```python
from build123d import *

# Parameters (mm, degrees)
BOSS_EXTRUDE1_DEPTH  = 2.7
SKETCH6_W            = 21.5
SKETCH6_H            = 36
BOSS_EXTRUDE2_DEPTH  = 2
SKETCH7_W            = 18.8
SKETCH7_H            = 11.32703558
CUT_EXTRUDE3_DEPTH   = 2
CUT_EXTRUDE4_DEPTH   = 41.5
SKETCH10_R           = 0.5
CUT_EXTRUDE5_DEPTH   = 41.5
CUT_EXTRUDE15_DEPTH  = 16
FILLET6_R            = 5
BOSS_EXTRUDE6_DEPTH  = 36
CUT_EXTRUDE18_DEPTH  = 1
CUT_EXTRUDE22_DEPTH  = 11.327036
CUT_EXTRUDE23_DEPTH  = 11.327036
BOSS_EXTRUDE10_DEPTH = 3
SKETCH43_W           = 2.3
SKETCH43_H           = 2.67296442
SKETCH43_H_2         = 8
SKETCH45_R           = 0.5
CUT_EXTRUDE26_DEPTH  = 38.82703558
SKETCH47_W           = 3.454078762
SKETCH47_H           = 22.63811533
CUT_EXTRUDE27_DEPTH  = 4
FILLET13_R           = 2
FILLET15_R           = 1
BOSS_EXTRUDE5_DEPTH  = 0.5
FILLET7_R            = 5


with BuildPart() as part:
    # Sketch3 → Boss-Extrude1 (new body)
    with BuildSketch(Plane(origin=(0, 0, 0), x_dir=(0, 0, -1), z_dir=(1, 0, 0))):
        with BuildLine():
            Line((0, 0), (45, 0))
            ThreePointArc((45, 0), (22.5, 6.928108612), (0, 0))
        make_face()
    extrude(amount=BOSS_EXTRUDE1_DEPTH)

    # Sketch6 → Boss-Extrude2 (add)
    with BuildSketch(Plane.XZ):
        with Locations((10.75, -22.5)):
            Rectangle(SKETCH6_W, SKETCH6_H)
    extrude(amount=BOSS_EXTRUDE2_DEPTH)

    # Sketch7 → Cut-Extrude3 (cut)
    with BuildSketch(Plane(origin=(0, 0, 0), x_dir=(1, 0, 0), z_dir=(0, 1, 0))):
        with Locations((12.1, 32.16351779)):
            Rectangle(SKETCH7_W, SKETCH7_H)
        with Locations((12.1, 12.83648221)):
            Rectangle(SKETCH7_W, SKETCH7_H)
    extrude(amount=-CUT_EXTRUDE3_DEPTH, mode=Mode.SUBTRACT)

    # Sketch8 → Cut-Extrude4 (cut, through all)
    with BuildSketch(Plane(origin=(0, 0, -40.5), x_dir=(-1, 0, 0), z_dir=(0, 0, -1))):
        with BuildLine():
            ThreePointArc((-21.5, -1), (-21.207106781, -0.292893219), (-20.5, 0))
            Line((-20.5, 0), (-21.5, 0))
            Line((-21.5, 0), (-21.5, -1))
        make_face()
        with BuildLine():
            ThreePointArc((-20.5, -2), (-21.207106781, -1.707106781), (-21.5, -1))
            Line((-21.5, -1), (-21.5, -2))
            Line((-21.5, -2), (-20.5, -2))
        make_face()
    extrude(amount=-CUT_EXTRUDE4_DEPTH, mode=Mode.SUBTRACT)

    # Sketch10 → Cut-Extrude5 (cut, through all)
    with BuildSketch(Plane(origin=(0, 0, -40.5), x_dir=(-1, 0, 0), z_dir=(0, 0, -1))):
        with Locations((-20.5, -1)):
            Circle(SKETCH10_R)
    extrude(amount=-CUT_EXTRUDE5_DEPTH, mode=Mode.SUBTRACT)

    # Sketch23 → Cut-Extrude15 (cut)
    with BuildSketch(Plane(origin=(0, 0, 0), x_dir=(1, 0, 0), z_dir=(0, 1, 0))):
        Polygon((11.878000054, 16.672665213), (21.5, 19.832983358), (21.5, 13.512347067), align=None)
        Polygon((21.5, 25.167016642), (21.5, 31.487652933), (11.878000054, 28.327334787), align=None)
    extrude(amount=-CUT_EXTRUDE15_DEPTH, mode=Mode.SUBTRACT)

    # Fillet6
    fillet6_edges = [part.edges().sort_by_distance(p)[0] for p in [
        (17.441558662, -1, -26.5),
        (17.441558662, -1, -18.5),
    ]]
    fillet(fillet6_edges, radius=FILLET6_R)

    # Sketch31 → Boss-Extrude6 (add)
    with BuildSketch(Plane(origin=(0, 0, -40.5), x_dir=(-1, 0, 0), z_dir=(0, 0, -1))):
        with BuildLine():
            Line((-14.656442534, -0.106610148), (-8.356442534, -0.106610148))
            ThreePointArc((-8.356442534, -0.106610148), (-11.506442534, -1.641351541), (-14.656442534, -0.106610148))
        make_face()
    extrude(amount=-BOSS_EXTRUDE6_DEPTH)

    # Sketch30 → Cut-Extrude18 (cut)
    with BuildSketch(Plane(origin=(0, 0, 0), x_dir=(1, 0, 0), z_dir=(0, 1, 0))):
        Polygon((17.131265183, 24.438450908), (4.7, 24.491454375), (4.7, 20.508545625), (17.131265183, 20.561549092), (18, 20.824521551), (18, 24.175478449), align=None)
    extrude(amount=-CUT_EXTRUDE18_DEPTH, mode=Mode.SUBTRACT)

    # Sketch36 → Cut-Extrude22 (cut)
    with BuildSketch(Plane.XY.offset(-37.82703558)):
        with BuildLine():
            Line((9.356442534, -0.106610148), (13.656442534, -0.106610148))
            ThreePointArc((13.656442534, -0.106610148), (11.506442534, -1.243174514), (9.356442534, -0.106610148))
        make_face()
    extrude(amount=CUT_EXTRUDE22_DEPTH, mode=Mode.SUBTRACT)

    # Sketch37 → Cut-Extrude23 (cut)
    with BuildSketch(Plane(origin=(0, 0, -7.17296442), x_dir=(-1, 0, 0), z_dir=(0, 0, -1))):
        with BuildLine():
            Line((-13.656442534, -0.106610148), (-9.356442534, -0.106610148))
            ThreePointArc((-9.356442534, -0.106610148), (-11.506442534, -1.243174514), (-13.656442534, -0.106610148))
        make_face()
    extrude(amount=CUT_EXTRUDE23_DEPTH, mode=Mode.SUBTRACT)

    # Sketch42 → Boss-Extrude10 (add)
    with BuildSketch(Plane.ZY):
        with BuildLine():
            Line((-45, 0), (-40.5, 0))
            Line((-40.5, 0), (-40.5, -2))
            Line((-40.5, -2), (-4.5, -2))
            Line((-4.5, -2), (-4.5, 0))
            Line((-4.5, 0), (0, 0))
            ThreePointArc((0, 0), (-22.5, 6.928108612), (-45, 0))
        make_face()
    extrude(amount=BOSS_EXTRUDE10_DEPTH)

    # Sketch43 → Cut-Revolve7 (revolve, cut)
    with BuildSketch(Plane.XZ.offset(2)):
        with Locations((-1.85, -5.83648221)):
            Rectangle(SKETCH43_W, SKETCH43_H)
        with Locations((-1.85, -22.5)):
            Rectangle(SKETCH43_W, SKETCH43_H_2)
        with Locations((-1.85, -39.16351779)):
            Rectangle(SKETCH43_W, SKETCH43_H)
    revolve(axis=Axis((-3, -2, -4.5), (0, 0, -1)), mode=Mode.SUBTRACT)

    # Sketch45 → Cut-Extrude26 (cut, through all)
    with BuildSketch(Plane.XY.offset(-7.17296442)):
        with Locations((-2, -1)):
            Circle(SKETCH45_R)
    extrude(amount=-CUT_EXTRUDE26_DEPTH, mode=Mode.SUBTRACT)

    # Sketch47 → Cut-Extrude27 (cut)
    with BuildSketch(Plane(origin=(0, 6.928108612, 0), x_dir=(1, 0, 0), z_dir=(0, 1, 0))):
        with Locations((-0.15, 22.5)):
            Rectangle(SKETCH47_W, SKETCH47_H)
    extrude(amount=-CUT_EXTRUDE27_DEPTH, mode=Mode.SUBTRACT)

    # Fillet13
    fillet13_edges = [part.edges().sort_by_distance(p)[0] for p in [
        (2.7, -2, -12.83648221),
        (2.7, -2, -32.16351779),
    ]]
    fillet(fillet13_edges, radius=FILLET13_R)

    # Fillet15
    fillet15_edges = [part.edges().sort_by_distance(p)[0] for p in [
        (-3, -2, -32.16351779),
        (-3, -2, -12.83648221),
    ]]
    fillet(fillet15_edges, radius=FILLET15_R)

    # Sketch27 → Boss-Extrude5 (add)
    with BuildSketch(Plane.XZ):
        Polygon((2.45, -4.5), (10, -4.5), (2.45, -2.5), align=None)
    extrude(amount=BOSS_EXTRUDE5_DEPTH)

    # Fillet7
    fillet7_edges = [part.edges().sort_by_distance(p)[0] for p in [
        (10, -0.25, -4.5),
    ]]
    fillet(fillet7_edges, radius=FILLET7_R)


solid = part.part
```
Build history of the part. All positions in model axes, mm. A direction names the side the tool comes from. Round coordinates to 2 decimals unless told otherwise and drop trailing zeros. Write each loop counter-clockwise with the first axis right and the second up, starting at its lowest first coordinate (ties: lowest second). Pieces come first, ordered by that corner, then holes.
1) Band-saw the part on B-B, the plane y = 5.75. List the corners of the cut face in (x, z), and give its area (3 significant figures).
2) 3-axis set-ups, long thin cutter, end or side, ignore diameter. For faces 5 (the cylindrical face through (11.471, -1.243, -12.757)), 6 (the cylindrical face through (-1.39, -0.36, -5.82)), 7 (the cylindrical face through (17.442, -1.014, -26.435)): which of +Z, -Z, +X, -X, +Y, -Y reach the whole face in a straight line?
3) Pin check, flat tips, straight feed: pin 1 (1.5 mm diameter, centred on y = 4.5, z = -14.5, fed in from +X); pin 2 (1.1 mm diameter, centred on x = 9, z = -33.5, fed in from +Y); pin 3 (1.2 mm diameter, centred on x = 10.5, z = -23, fed in from +Y). Stop position of each tip, or through.
4) Mould opens along X. For faces 1 (the cylindrical face through (20, -1, -39)), 2 (the cylindrical face through (-1.39, -0.36, -39.14)), 3 (the flat face through (7, -2, -23)), 4 (the flat face through (0, 2.928, -23)) say: +X half, -X half, draft (parallel to the pull), parting line (faces both ways), or undercut.
5) Band-saw the part on C-C, the plane x = 5.5. List the corners of the cut face in (y, z), and give its area (3 significant figures).
6) Drill centre lines: probe 1 along Y at (x, z) = (20.5, -21.5); probe 2 along X at (y, z) = (4.5, -12); probe 3 along X at (y, z) = (1.5, -10). Where is each one in solid material? Low to high.
7) Band-saw the part on D-D, the plane z = -15.5. Give the number of separate pieces and of enclosed holes in the cut face, and give its area (3 significant figures).
8) Band-saw the part on A-A, the plane x = 0.25. List the corners of the cut face in (y, z), and give its area (3 significant figures).
Ans:
1. outline: (-3, -32.14) - (-1.88, -32.14) - (-1.88, -12.86) - (-3, -12.86) - close; (1.58, -32.14) - (2.7, -32.14) - (2.7, -12.86) - (1.58, -12.86) - close
1. area: 43.3 mm2
2. face 5: +Y
2. face 6: -X, -Y
2. face 7: +X, +Y, -Y
3. pin 1: stops at x = 2.7
3. pin 2: stops at y = -0.11
3. pin 3: stops at y = -1
4. face 1: undercut
4. face 2: -X half
4. face 3: draft
4. face 4: undercut
5. outline: (-2, -40.5) - (0, -40.5) - (0, -37.83) - (-2, -37.83) - close; (-2, -26.5) - (0, -26.5) - (0, -24.49) - (-1, -24.49) - (-1, -20.51) - (0, -20.51) - (0, -18.5) - (-2, -18.5) - close; (-2, -7.17) - (0, -7.17) - (0, -3.31) - (-0.5, -3.31) - (-0.5, -4.5) - (-2, -4.5) - close
5. area: 23.3 mm2
6. probe 1: y = -2 to -1.5, -0.5 to 0
6. probe 2: x = -3 to -1.88, 1.58 to 2.7
6. probe 3: x = -3 to 2.7
7. separate pieces: 2
7. enclosed holes: 1
7. area: 37.1 mm2
8. outline: (-2, -40.5) - (0, -40.5) - (0, -45) arc R40 ccw to (5.29, -33.82) - (2.93, -33.82) - (2.93, -11.18) - (5.29, -11.18) arc R40 ccw to (0, 0) - (0, -4.5) - (-2, -4.5) - close
8. area: 205 mm2
